Part model, mm, in its own coordinate system. A direction names the side the tool comes from. Round coordinates to 2 decimals unless told otherwise and drop trailing zeros. Write each loop counter-clockwise with the first axis right and the second up, starting at its lowest first coordinate (ties: lowest second). Pieces come first, ordered by that corner, then holes.
1) Which spindle directions (+Z, -Z, +X, -X, +Y, -Y) get a long thin tool onto all of the face, cutting with end or side? Do faces 5 (the flat face through (65.216, -1, 11)), 6 (the cylindrical face through (20.913, -56.95, 12.423)), 7 (the flat face through (-21, 56.304, 11)), 8 (the cylindrical face through (21.14, 56.95, 11.91)). Say none if no direction does.
2) Drill centre lines: L1, parallel to Y at x = -48.5, z = 6; L2, parallel to Y at x = -5, z = 27.3; L3, parallel to X at y = -4, z = 9. Where is each one in solid material? Low to high.
3) Saw through at C-C on y = -38.5. Write the cut outline in (x, z), and give its area (3 significant figures).
4) Saw through at B-B on z = 6.5. Write the cut outline in (x, y), and give its area (3 significant figures).
5) Saw through at D-D on x = 37.5. Write the cut outline in (y, z), and give its area (3 significant figures).
6) Flat gauge pins, fed straight in: pin 1 (4 mm diameter, centred on x = -5, y = -46.23, fed in from -Z); pin 2 (1.6 mm diameter, centred on x = 66, z = 9.5, fed in from -Y); pin 3 (2 mm diameter, centred on x = 66.5, z = -0.5, fed in from +Y); pin 4 (2.5 mm diameter, centred on x = -5, y = 48.27, fed in from -Z). Where does each tip first touch, or does it go through?
7) Saw through at A-A on x = -5. Write the cut outline in (y, z), and give its area (3 significant figures).
8) Pull direction X, two halves, no side cores. Call faces 1 (the flat face through (67.216, -1, 12)), 2 (the flat face through (-65.216, -1, 11)), 3 (the flat face through (-21.324, -56.783, 27.521)), 4 (the flat face through (-1, 1, 27)): +X half, -X half, draft (parallel to the pull), parting line (faces both ways), or undercut.
```python
from build123d import *

# Parameters (mm, degrees)
SKETCH008_W      = 134.431716
SKETCH008_H      = 116.608648
PAD008_DEPTH     = 34
THICKNESS_T      = -2
HOLE_D           = 3
HOLE_DEPTH       = 25
HOLE_CSINK_D     = 4.5
HOLE_CSINK_ANGLE = 90
HOLE_TIPS_R      = 1.5
SKETCH011_W      = 22.22
SKETCH011_H      = 30.19
SKETCH011_W_2    = 21.462421
SKETCH011_H_2    = 8.812902
POCKET_DEPTH     = 5
SKETCH012_R      = 36
POCKET001_DEPTH  = 5
SKETCH013_R      = 36
POCKET002_DEPTH  = 5
CHAMFER_SIZE     = 3
SKETCH015_W      = 11.6
SKETCH015_H      = 20.6
POCKET003_DEPTH  = 5
CHAMFER001_SIZE  = 1


with BuildPart() as part:
    # Sketch008 → Pad008 (new body)
    with BuildSketch(Plane.XY):
        Rectangle(SKETCH008_W, SKETCH008_H)
    extrude(amount=PAD008_DEPTH)

    # Thickness
    thickness_openings = [part.faces().sort_by_distance(p)[0] for p in [
        (0, 0, 0),
    ]]
    offset(amount=THICKNESS_T, openings=thickness_openings)

    # Hole
    with Locations(Plane.XY.offset(34)):
        with Locations((-5, 48.267742), (-5, -46.232258)):
            CounterSinkHole(HOLE_D / 2, HOLE_CSINK_D / 2, depth=HOLE_DEPTH, counter_sink_angle=HOLE_CSINK_ANGLE)

    # Hole tips → Hole tip 1 section 0
    with BuildSketch(Plane.XY.offset(9), mode=Mode.PRIVATE) as hole_tip_1_s0:
        with Locations((-5, 48.267742)):
            Circle(HOLE_TIPS_R)
    loft([hole_tip_1_s0.sketch, Vertex(-5, 48.267742, 8.098709)], mode=Mode.SUBTRACT)

    # Hole tips → Hole tip 2 section 0
    with BuildSketch(Plane.XY.offset(9), mode=Mode.PRIVATE) as hole_tip_2_s0:
        with Locations((-5, -46.232258)):
            Circle(HOLE_TIPS_R)
    loft([hole_tip_2_s0.sketch, Vertex(-5, -46.232258, 8.098709)], mode=Mode.SUBTRACT)

    # Sketch011 (on Face3 of Hole) → Pocket (cut)
    with BuildSketch(Plane.YZ.offset(67.215858)):
        with Locations((43.25677, 15.095)):
            Rectangle(SKETCH011_W, SKETCH011_H)
        with Locations((-42.456113, 15.095)):
            Rectangle(SKETCH011_W, SKETCH011_H)
        with Locations((-1.636131, 4.406451)):
            Rectangle(SKETCH011_W_2, SKETCH011_H_2)
    extrude(amount=-POCKET_DEPTH, mode=Mode.SUBTRACT)

    # Sketch012 (on Face1 of Pocket) → Pocket001 (cut)
    with BuildSketch(Plane(origin=(0, 58.304324, 0), x_dir=(-1, 0, 0), z_dir=(0, 1, 0))):
        with Locations((-57.121563, 15.810025)):
            Circle(SKETCH012_R)
    extrude(amount=-POCKET001_DEPTH, mode=Mode.SUBTRACT)

    # Sketch013 (on Face13 of Pocket001) → Pocket002 (cut)
    with BuildSketch(Plane.XZ.offset(58.304324)):
        with Locations((56.871254, 15.696718)):
            Circle(SKETCH013_R)
    extrude(amount=-POCKET002_DEPTH, mode=Mode.SUBTRACT)

    # Chamfer
    chamfer_edges = [part.edges().sort_by_distance(p)[0] for p in [
        (-20.67222, -58.304324, 34),
        (-67.215858, 0, 34),
        (-20.580376, 58.304324, 34),
    ]]
    chamfer(chamfer_edges, length=CHAMFER_SIZE)

    # Sketch015 (on Face1 of Chamfer) → Pocket003 (cut)
    with BuildSketch(Plane(origin=(0, 58.304324, 0), x_dir=(-1, 0, 0), z_dir=(0, 1, 0))):
        with Locations((5.414926, 17.771388)):
            Rectangle(SKETCH015_W, SKETCH015_H)
    extrude(amount=-POCKET003_DEPTH, mode=Mode.SUBTRACT)

    # Chamfer001
    chamfer001_edges = [part.edges().sort_by_distance(p)[0] for p in [
        (66.215858, -31.346113, 0),
        (66.215858, -31.346113, 30.19),
        (66.215858, 9.09508, 8.812902),
        (66.215858, 9.09508, 0),
    ]]
    chamfer(chamfer001_edges, length=CHAMFER001_SIZE)


with BuildPart() as part_1:
    # Body001 placement: moved
    add(part.part.moved(Location((0, 0, -5))))


solid = part_1.part
```
Completed:
1. face 5: -Z, +Y, -Y
1. face 6: +X, -Y
1. face 7: -Z, +X
1. face 8: +X, +Y
2. L1: y = -58.3 to -56.3, 56.3 to 58.3
2. L2: y = -57 to -47.73, -44.73 to 46.77, 49.77 to 57
2. L3: x = -67.22 to -65.22, 65.22 to 67.22
3. outline: (-67.22, -5) - (-65.22, -5) - (-65.22, 27) - (65.22, 27) - (65.22, 25.19) - (67.22, 25.19) - (67.22, 29) - (-64.22, 29) - (-67.22, 26) - close
3. area: 332 mm2
4. outline: (-67.22, -58.3) - (21.12, -58.3) - (21.12, -56.3) - (-65.22, -56.3) - (-65.22, 56.3) - (-11.21, 56.3) - (-11.21, 58.3) - (-67.22, 58.3) - close; (0.39, 56.3) - (21.38, 56.3) - (21.38, 58.3) - (0.39, 58.3) - close; (65.22, -31.35) - (67.22, -31.35) - (67.22, 32.15) - (65.22, 32.15) - close
4. area: 683 mm2
5. outline: (-53.3, 27) - (53.3, 27) - (53.3, 29) - (-53.3, 29) - close
5. area: 213 mm2
6. pin 1: stops at z = 27
6. pin 2: stops at y = -31.35
6. pin 3: stops at y = 32.15
6. pin 4: passes through
7. outline: (-58.3, -5) - (-56.3, -5) - (-56.3, 27) - (-47.73, 27) - (-47.73, 28.25) - (-48.48, 29) - (-55.3, 29) - (-58.3, 26) - close; (-44.73, 27) - (46.77, 27) - (46.77, 28.25) - (46.02, 29) - (-43.98, 29) - (-44.73, 28.25) - close; (49.77, 27) - (56.3, 27) - (56.3, 23.07) - (58.3, 23.07) - (58.3, 26) - (55.3, 29) - (50.52, 29) - (49.77, 28.25) - close; (56.3, -5) - (58.3, -5) - (58.3, 2.47) - (56.3, 2.47) - close
7. area: 298 mm2
8. face 1: +X half
8. face 2: undercut
8. face 3: draft
8. face 4: undercut
